For this review, take the finished solid that the model builds, in its own axes (mm). A direction names the side the tool comes from. Give positions to 0.01 mm unless a question says otherwise; leave off trailing zeros. Write each loop counter-clockwise with the first axis right and the second up, starting at its lowest first coordinate (ties: lowest second). Pieces come first, ordered by that corner, then holes. Notation, with made-up numbers: M -7.5,68 L 36.5,68 A17 ccw 36.5,82 Z; hole C 36,-14 d7. An arc over 180 degrees is marked long. Answer as a JSON object with one key per item and string values. Group by question number.
```python
from build123d import *

# Parameters (mm, degrees)
PAD_DEPTH    = 8
PAD001_DEPTH = 16
PAD002_DEPTH = 8
SKETCH004_R  = 11
PAD003_DEPTH = 2
SKETCH005_R  = 2.5
PAD004_DEPTH = 16
SKETCH006_R  = 1.5
POCKET_DEPTH = 5


with BuildPart() as part:
    # Sketch → Pad (new body)
    with BuildSketch(Plane.XY):
        Polygon((4.5, -4.5), (37.5, -4.5), (42, 0), (42, 33), (37.5, 37.5), (4.5, 37.5), (0, 33), (0, 0), align=None)
    extrude(amount=PAD_DEPTH)

    # Sketch002 (on Face10 of Pad) → Pad001 (join)
    with BuildSketch(Plane.XY.offset(8)):
        Polygon((7.5, 37.5), (34.5, 37.5), (42, 30), (42, 3), (34.5, -4.5), (7.5, -4.5), (0, 3), (0, 30), align=None)
    extrude(amount=PAD001_DEPTH)

    # Sketch003 (on Face15 of Pad001) → Pad002 (join)
    with BuildSketch(Plane.XY.offset(24)):
        Polygon((4.5, 37.5), (37.5, 37.5), (42, 33), (42, 0), (37.5, -4.5), (4.5, -4.5), (0, 0), (0, 33), align=None)
    extrude(amount=PAD002_DEPTH)

    # Sketch004 (on Face7 of Pad002) → Pad003 (join)
    with BuildSketch(Plane.XY.offset(32)):
        with Locations((21.15, 16.65)):
            Circle(SKETCH004_R)
    extrude(amount=PAD003_DEPTH)

    # Sketch005 (on Face27 of Pad003) → Pad004 (join)
    with BuildSketch(Plane.XY.offset(34)):
        with Locations((21.15, 16.65)):
            Circle(SKETCH005_R)
    extrude(amount=PAD004_DEPTH)

    # Sketch006 (on Face7 of Pad004) → Pocket (cut)
    with BuildSketch(Plane.XY.offset(32)):
        with Locations((5.65, 1.15)):
            Circle(SKETCH006_R)
        with Locations((36.65, 1.15)):
            Circle(SKETCH006_R)
        with Locations((36.65, 32.15)):
            Circle(SKETCH006_R)
        with Locations((5.65, 32.15)):
            Circle(SKETCH006_R)
    extrude(amount=-POCKET_DEPTH, mode=Mode.SUBTRACT)


with BuildPart() as part_1:
    # Body placement: moved
    add(part.part.moved(Location((-21.15, -16.65, -57.5))))


solid = part_1.part
```
Item 1: To check wall thickness, follow probe 1 along Y at (x, z) = (-15.5, -27.9); probe 2 along Y at (x, z) = (-15, -27); probe 3 along Z at (x, y) = (-1.5, 4.5). State the ranges of each line that lie inside material, in increasing order.
Item 2: Consider section A-A (z = -28). Give the boundary of the cut face in (x, y).
Item 3: Consider section C-C (y = 0). Give the boundary of the cut face in (x, z), plus the area to 3 significant figures.
Item 4: Consider section D-D (z = -36). Give the boundary of the cut face in (x, y), plus the area to 3 significant figures.
Item 5: Insertion check: P1, Ø6, axis at x = 15.5, y = 18, coming from the +Z side; P2, Ø2.5, axis at x = 15.5, y = -15.5, coming from the +Z side; P3, Ø8, axis at x = -11, y = 6.5, coming from the +Z side. Each pin has a flat end and moves straight along its axis. Give the tip position at first contact, or say it passes through.
Item 6: Machinability: for faces 4 (the flat face through (-16, -15, -30.5)), 5 (the flat face through (18, 18, -33.5)), 6 (the flat face through (17.2, -17.3, -41.6)), 7 (the flat face through (-18, 18, -49.5)), which of the approach directions +Z, -Z, +X, -X, +Y, -Y give a long, thin tool a straight path to every point of the face, cutting with its end or side? Answer none if there is none.
Item 7: Consider section B-B (x = -15.5). Give the boundary of the cut face in (y, z), plus the area to 3 significant figures.
Item 8: Draft analysis for pull direction Y (two halves, no side actions). For faces 1 (the cylindrical face through (-16.7, -16.4, -28)), 2 (the flat face through (-18.9, 18.6, -53.6)), 3 (the flat face through (-18, 18, -33.5)), state which applies: released by +Y, released by -Y, zero draft, split by the parting line, or undercut.
Result set:
{
 "1": {"probe 1": "y = -21.15 to -17, -14 to 14, 17 to 20.85", "probe 2": "y = -21.15 to -16.91, -14.09 to 14.09, 16.91 to 20.85", "probe 3": "z = -57.5 to -23.5"},
 "2": {"outline": "M -21.15,-16.65 L -16.65,-21.15 L 16.35,-21.15 L 20.85,-16.65 L 20.85,16.35 L 16.35,20.85 L -16.65,20.85 L -21.15,16.35 Z; hole C -15.5,-15.5 d3; hole C -15.5,15.5 d3; hole C 15.5,-15.5 d3; hole C 15.5,15.5 d3"},
 "3": {"outline": "M -21.15,-57.5 L 20.85,-57.5 L 20.85,-25.5 L 11,-25.5 L 11,-23.5 L 2.5,-23.5 L 2.5,-7.5 L -2.5,-7.5 L -2.5,-23.5 L -11,-23.5 L -11,-25.5 L -21.15,-25.5 Z", "area": "1,470 mm^2"},
 "4": {"outline": "M -21.15,-13.65 L -13.65,-21.15 L 13.35,-21.15 L 20.85,-13.65 L 20.85,13.35 L 13.35,20.85 L -13.65,20.85 L -21.15,13.35 Z", "area": "1,650 mm^2"},
 "5": {"P1": "stops at z = -25.5", "P2": "stops at z = -30.5", "P3": "stops at z = -23.5"},
 "6": {"face 4": "+Z", "face 5": "+X, +Y", "face 6": "+X, -Y", "face 7": "-X, +Y"},
 "7": {"outline": "M -21.15,-57.5 L 20.85,-57.5 L 20.85,-49.5 L 19,-49.5 L 19,-33.5 L 20.85,-33.5 L 20.85,-25.5 L 17,-25.5 L 17,-30.5 L 14,-30.5 L 14,-25.5 L -14,-25.5 L -14,-30.5 L -17,-30.5 L -17,-25.5 L -21.15,-25.5 L -21.15,-33.5 L -19.3,-33.5 L -19.3,-49.5 L -21.15,-49.5 Z", "area": "1,250 mm^2"},
 "8": {"face 1": "undercut", "face 2": "released by +Y", "face 3": "zero draft"}
}
